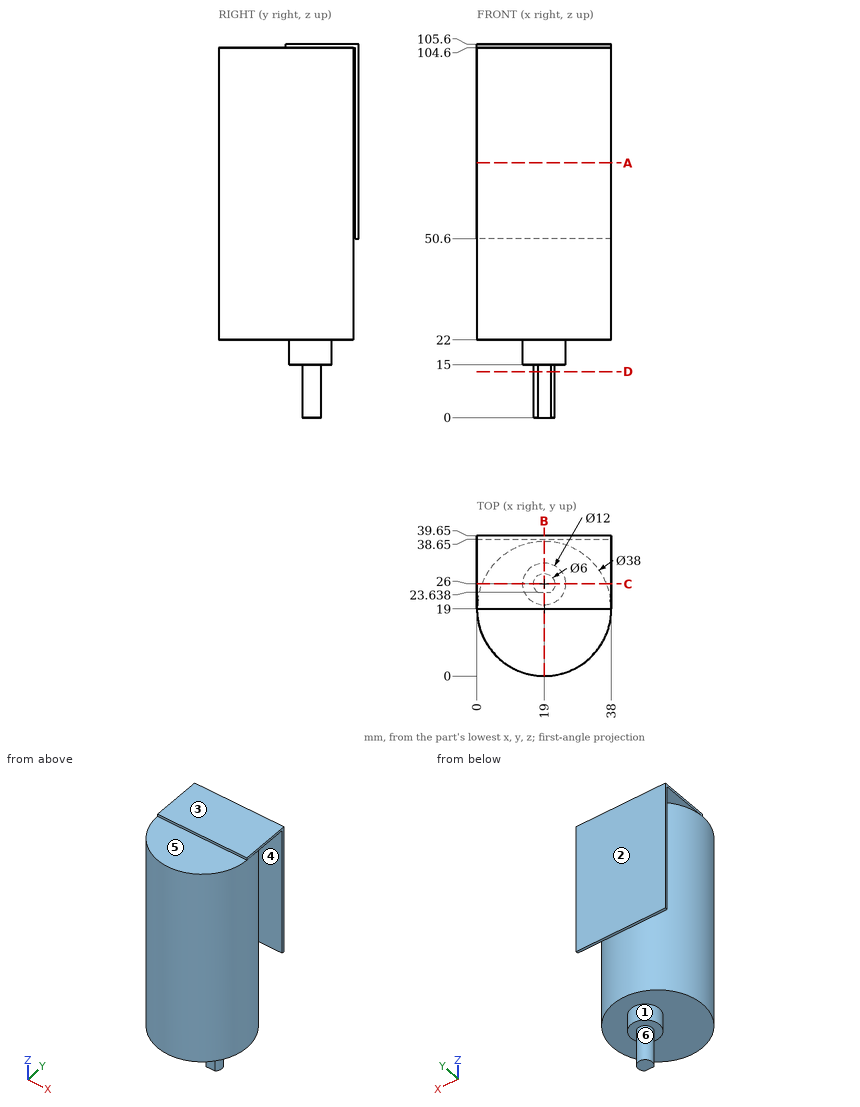
Geometry: see drawing. Coordinates: mm, zero at the bounding-box minimum. A direction names the side the tool comes from. Round coordinates to 2 decimals unless told otherwise and drop trailing zeros. Write each loop counter-clockwise with the first axis right and the second up, starting at its lowest first coordinate (ties: lowest second). Pieces come first, ordered by that corner, then holes.
Item 1: Section query B-B (x = 19). Return loops of the section in (y, z).
Item 2: Mould query, pull axis Y, two halves, no side actions, for the marked faces 1, 2, 3 and 4. Classes: +Y half, -Y half, draft (parallel to the pull), parting line (faces both ways), or undercut.
Item 3: Pin query (flat end, axial travel): P1, Ø2, axis at x = 16.5, z = 92.5, coming from the -Y side; P2, Ø1.5, axis at x = 23.5, y = 18.5, coming from the -Z side; P3, Ø21, axis at x = 10, y = 7, coming from the +Z side. Return the tip coordinate at first contact, or that it passes through.
Item 4: Set-up query: the marked faces 5 and 6. Return all of +Z, -Z, +X, -X, +Y, -Y with unobstructed straight access to the full face (end or side cutting, diameter ignored); none if empty.
Item 5: Section query A-A (z = 72). Return loops of the section in (x, y), plus the area to 3 significant figures.
Item 6: Section query D-D (z = 13). Return loops of the section in (x, y), plus the area to 3 significant figures.
Item 7: Section query C-C (y = 26). Return loops of the section in (x, z), plus the area to 3 significant figures.
Item 8: Material intervals for L1, parallel to Z at x = 4, y = 34; L2, parallel to Z at x = 33, y = 21; L3, parallel to Y at x = 27, z = 100.5, sorted ascending.
Completed:
1. outline: (0, 22) - (20, 22) - (20, 15) - (23.64, 15) - (23.64, 0) - (29, 0) - (29, 15) - (32, 15) - (32, 22) - (38, 22) - (38, 104.6) - (38.65, 104.6) - (38.65, 50.6) - (39.65, 50.6) - (39.65, 105.6) - (19, 105.6) - (19, 104.6) - (0, 104.6) - close
2. face 1: parting line
2. face 2: +Y half
2. face 3: draft
2. face 4: undercut
3. P1: stops at y = 0.06
3. P2: stops at z = 22
3. P3: stops at z = 104.6
4. face 5: +Z, +X, -X, -Y
4. face 6: -Z
5. outline: circle Ø38 at (19, 19); (0, 38.65) - (38, 38.65) - (38, 39.65) - (0, 39.65) - close
5. area: 1,170 mm2
6. outline: (17.15, 23.64) - (20.85, 23.64) arc R3 ccw (long way) to start
6. area: 26.7 mm2
7. outline: (0, 104.6) - (1.34, 104.6) - (1.34, 22) - (13, 22) - (13, 15) - (16, 15) - (16, 0) - (22, 0) - (22, 15) - (25, 15) - (25, 22) - (36.66, 22) - (36.66, 104.6) - (38, 104.6) - (38, 105.6) - (0, 105.6) - close
7. area: 3,130 mm2
8. L1: z = 104.6 to 105.6
8. L2: z = 22 to 105.6
8. L3: y = 1.77 to 36.23, 38.65 to 39.65
